The listing builds one solid part. Answer for the finished solid, in the listing's coordinates (mm). A direction names the side the tool comes from. Coordinates: 2 decimals unless noted, no trailing zeros. Order: outer loops, then holes, each group sorted by start corner. A loop starts at its lowest first (then second) coordinate and runs counter-clockwise, first axis right, second up. Notation, with made-up numbers: M -3.5,87.25 L 6.5,87.25 A4 cw 6.5,94.25 Z; hole C 83,71.5 d7. An arc over 180 degrees is marked long. One line per item, written item: value. Start each with the question number.
Q1. The part is cut by section A-A on x = 7. Give the vertices of the cut face in (y, z), then the cut area to 3 significant figures.
Q2. Straight lines are drawn through the part: line 1 along X through (y, z) = (1.5, 4); line 2 along X through (y, z) = (0.5, 4); line 3 along Z through (x, y) = (15.5, 0). For each, find the intervals that lie inside material, in ascending order. Write a range as [from, to].
Q3. Determine the mould class of faces 4 (the cylindrical face through (7.46, 5.39, -1.7)), 5 (the conical face through (-14.248, 1.19, 0.733)), 6 (the conical face through (24.63, -7.52, -0.09)), 7 (the conical face through (20.404, 7.309, -0.074)) for opening direction Y: pulls with the +Y half, pulls with the -Y half, needs draft (parallel to the pull), parting line crosses it, or undercut.
Q4. The part is cut by section B-B on x = -1. Give the vertices of the cut face in (y, z).
Q5. Each of these flat-tipped pins is pushed along its axis until it touches: pin 1 Ø5 at (x, y) = (8, -5) entering from -Z; pin 2 Ø2 at (x, z) = (4.5, -3) entering from -Y; pin 3 Ø6 at (x, y) = (24.5, 2) entering from +Z. Where does it stop, or does it pass through?
Q6. The part is cut by section C-C on x = 23.5. Give the vertices of the cut face in (y, z), then the cut area to 3 significant figures.
Q7. For faces 1 (the conical face through (20.404, -7.309, 0.074)), 2 (the flat face through (10.3, -5, 1)), 3 (the flat face through (25.9, 0, 0)), determine the directions among +Z, -Z, +X, -X, +Y, -Y from which every point of the face is accessible in a straight line to the end or side of a thin tool.
Autodesk Inventor part; units mm, degrees
ref_plane "Work Plane1" through (0, 4.9, 0) normal (0, 1, 0) x (-1, 0, 0)
ref_plane "Work Plane2" through (0, 0, 5) normal (0, 0, 1) x (1, 0, 0)
ref_plane "YZ Plane" through (0, 0, 0) normal (1, 0, 0) x (0, 1, 0)
sketch "Sketch1" plane through (0, 0, 0) normal (0, 0, 1) x (1, 0, 0)
  line L0 (25.9, 0) -> (25.9, 6.25)
  line L1 (22.7, 9.45) -> (20.3, 9.45)
  line L2 (20.3, 9.45) -> (20.3, 7.175) construction
  line L3 (20.3, 4.7) -> (10.3, 4.7)
  line L4 (10.3, 4.7) -> (10.3, 5.65)
  line L5 (10.3, 5.65) -> (4.7, 5.65)
  line L6 (4.7, 5.65) -> (4.7, 4.7)
  line L7 (4.7, 4.7) -> (-23.9, 4.7)
  line L8 (-25.9, 2.7) -> (-25.9, 0)
  line L9 (-25.9, 0) -> (25.9, 0)
  line L10 (-23.9, 4.7) -> (-25.9, 2.7)
  line L11 (25.9, 6.25) -> (22.7, 9.45)
  line L12 (20.3, 9.45) -> (20.9, 7.95)
  line L13 (20.9, 7.95) -> (20.3, 7.175)
  line L14 (20.3, 7.175) -> (20.9, 5.95)
  line L15 (20.9, 5.95) -> (20.3, 5.1)
  line L16 (20.3, 7.175) -> (20.3, 5.1) construction
  line L17 (20.3, 5.1) -> (20.3, 4.7)
  point P0 (0, 0)
  point P1 (25.9, 9.45)
  point P2 (-25.9, 4.7)
  point P3 (0, 0)
  dimension "d0" = 9.45
  dimension "d1" = 5.6
  dimension "d2" = 51.8
  dimension "d3" = 4.7
  dimension "d4" = 10
  dimension "d5" = 5.6
  dimension "d6" = 5.65
  dimension "d7" = 2
  dimension "d8" = 2
  dimension "d10" = 3.2
  dimension "d11" = 3.2
  dimension "d26" = 0.6
  dimension "d27" = 1.5
  dimension "d28" = 2
  dimension "d29" = 0.4
  dimension "d30" = 2.275
revolve "Revolution1" add sketch "Sketch1" angle 360 about axis through (-25.9, 0, 0) along (1, 0, 0)
sketch "Sketch2" plane through (25.9, 0, 0) normal (1, 0, 0) x (0, 0, -1)
  line L0 (-4.75, 9.5) -> (4.75, 9.5) construction
  line L1 (4.75, 9.5) -> (4.75, -9.5)
  line L2 (4.75, -9.5) -> (-4.75, -9.5) construction
  line L3 (-4.75, -9.5) -> (-4.75, 9.5)
  line L4 (4.75, 9.5) -> (9.75, 9.5)
  line L5 (9.75, 9.5) -> (9.75, -9.5)
  line L6 (9.75, -9.5) -> (4.75, -9.5)
  line L7 (-4.75, 9.5) -> (-9.75, 9.5)
  line L8 (-9.75, 9.5) -> (-9.75, -9.5)
  line L9 (-9.75, -9.5) -> (-4.75, -9.5)
  point P0 (0, 0)
  point P1 (0, 9.5)
  point P2 (-4.75, 0)
  dimension "d12" = 9.5
  dimension "d13" = 19
  dimension "d14" = 5
extrude "Extrusion1" cut sketch "Sketch2" against normal blind 5.8
ref_plane "Work Plane1" through (0, 4.9, 0) normal (0, 1, 0) x (-1, 0, 0)
sketch "Sketch3" plane through (0, 4.9, 0) normal (0, 1, 0) x (-1, 0, 0)
  line L0 (-4.7, 5.65) -> (-4.7, -5.65)
  point P0 (0, 0)
  point P1 (14.3, 0)
  dimension "d18" = 19
hole "0°" [suppressed]
ref_plane "Work Plane2" through (0, 0, 5) normal (0, 0, 1) x (1, 0, 0)
sketch "Sketch4" plane through (0, 0, 5) normal (0, 0, 1) x (1, 0, 0)
  line L0 (4.7, -5.65) -> (4.7, 5.65)
  point P0 (0, 0)
  point P1 (-14.3, 0)
  dimension "d32" = 19
hole "90°" at (-14.3, 0, 5) direction (0, 0, -1) diameter 14 depth 0.2 tip angle 110
properties part number "Tornillo en T esquinero"
Output:
1. outline: C 0,0 d11.3
1. area: 100 mm^2
2. line 1: x = [-24.33, -19.96], [-8.64, 25.9]
2. line 2: x = [-24.57, -20.14], [-8.46, 25.9]
2. line 3: z = [-4.7, 4.7]
3. face 4: parting line crosses it
3. face 5: undercut
3. face 6: pulls with the -Y half
3. face 7: undercut
4. outline: C 0,0 d9.4
5. pin 1: stops at z = -5.07
5. pin 2: stops at y = -5.28
5. pin 3: stops at z = 4.75
6. outline: M -7.23,-4.75 L 7.23,-4.75 A8.65 ccw 7.23,4.75 L -7.23,4.75 A8.65 ccw Z
6. area: 156 mm^2
7. face 1: -X
7. face 2: none
7. face 3: +Z, -Z, +X, +Y, -Y
